Can you work these out from the model? Positions are in its coordinate system, mm. Round coordinates to 2 decimals unless told otherwise and drop trailing zeros. Loops run counter-clockwise (first coordinate to the right, second up) from the corner with the lowest first, then second, coordinate; pieces in that order, holes last. Notation, with made-up numbers: (-37.75, -37.75) -> (-5.75, -37.75) arc R30 ccw to (-5.75, -6.75) -> close; hole circle Ø11 at (47, -12). An arc over 180 degrees is marked (long way). Use a Markdown table: item, result.
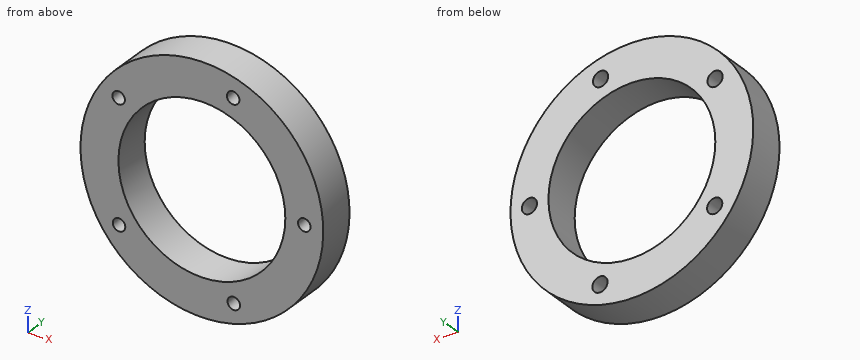
from build123d import *

# Parameters (mm, degrees)
SKETCH1_R                    = 16
SKETCH1_R_2                  = 11
BOSS_EXTRUDE2_DEPTH          = 5
SKETCH2_R                    = 1
CUT_EXTRUDE1_DEPTH           = 5
CUT_EXTRUDE1_DRAFT           = -2
CUT_EXTRUDE1_PROFILE_2_DEPTH = 5
CUT_EXTRUDE1_PROFILE_2_DRAFT = -2
CUT_EXTRUDE1_PROFILE_3_DEPTH = 5
CUT_EXTRUDE1_PROFILE_3_DRAFT = -2
CUT_EXTRUDE1_PROFILE_4_DEPTH = 5
CUT_EXTRUDE1_PROFILE_4_DRAFT = -2
CUT_EXTRUDE1_PROFILE_5_DEPTH = 5
CUT_EXTRUDE1_PROFILE_5_DRAFT = -2


with BuildPart() as part:
    # Sketch1 → Boss-Extrude2 (new body)
    with BuildSketch(Plane(origin=(0, 0, 0), x_dir=(1, 0, 0), z_dir=(0, 1, 0))):
        with Locations(Location((0, 0, 0), (0, 0, 270))):
            Circle(SKETCH1_R)
        with Locations(Location((0, 0, 0), (0, 0, 270))):
            Circle(SKETCH1_R_2, mode=Mode.SUBTRACT)
    extrude(amount=BOSS_EXTRUDE2_DEPTH)


with BuildPart() as cut_extrude1_tool:
    # Sketch2 → Cut-Extrude1 (with draft: the straight prism first)
    with BuildSketch(Plane(origin=(0, 5, 0), x_dir=(1, 0, 0), z_dir=(0, 1, 0))):
        with Locations((-10.918529424, 8.01503688)):
            Circle(SKETCH2_R)
    extrude(amount=-CUT_EXTRUDE1_DEPTH)
    # Cut-Extrude1: the draft: its side faces are tilted about the plane it starts from
    cut_extrude1_sides = [cut_extrude1_tool.faces().sort_by_distance(p)[0] for p in [
        (-11.918529424, 2.5, -8.01503688),
    ]]
    draft(cut_extrude1_sides, Plane(origin=(0, 5, 0), x_dir=(1, 0, 0), z_dir=(0, 1, 0)), CUT_EXTRUDE1_DRAFT)


with BuildPart() as part_1:
    add(part.part)

    # Cut-Extrude1: cut by cut_extrude1_tool
    add(cut_extrude1_tool.part, mode=Mode.SUBTRACT)


with BuildPart() as cut_extrude1_profile_2_tool:
    # Sketch2 → Cut-Extrude1 profile 2 (with draft: the straight prism first)
    with BuildSketch(Plane(origin=(0, 5, 0), x_dir=(1, 0, 0), z_dir=(0, 1, 0))):
        with Locations((-10.966125757, -7.868550431)):
            Circle(SKETCH2_R)
    extrude(amount=-CUT_EXTRUDE1_PROFILE_2_DEPTH)
    # Cut-Extrude1 profile 2: the draft: its side faces are tilted about the plane it starts from
    cut_extrude1_profile_2_sides = [cut_extrude1_profile_2_tool.faces().sort_by_distance(p)[0] for p in [
        (-11.966125757, 2.5, 7.868550431),
    ]]
    draft(cut_extrude1_profile_2_sides, Plane(origin=(0, 5, 0), x_dir=(1, 0, 0), z_dir=(0, 1, 0)), CUT_EXTRUDE1_PROFILE_2_DRAFT)


with BuildPart() as part_2:
    add(part_1.part)

    # Cut-Extrude1 profile 2: cut by cut_extrude1_profile_2_tool
    add(cut_extrude1_profile_2_tool.part, mode=Mode.SUBTRACT)


with BuildPart() as cut_extrude1_profile_3_tool:
    # Sketch2 → Cut-Extrude1 profile 3 (with draft: the straight prism first)
    with BuildSketch(Plane(origin=(0, 5, 0), x_dir=(1, 0, 0), z_dir=(0, 1, 0))):
        with Locations((4.125355383, -12.822115645)):
            Circle(SKETCH2_R)
    extrude(amount=-CUT_EXTRUDE1_PROFILE_3_DEPTH)
    # Cut-Extrude1 profile 3: the draft: its side faces are tilted about the plane it starts from
    cut_extrude1_profile_3_sides = [cut_extrude1_profile_3_tool.faces().sort_by_distance(p)[0] for p in [
        (3.125355383, 2.5, 12.822115645),
    ]]
    draft(cut_extrude1_profile_3_sides, Plane(origin=(0, 5, 0), x_dir=(1, 0, 0), z_dir=(0, 1, 0)), CUT_EXTRUDE1_PROFILE_3_DRAFT)


with BuildPart() as part_3:
    add(part_2.part)

    # Cut-Extrude1 profile 3: cut by cut_extrude1_profile_3_tool
    add(cut_extrude1_profile_3_tool.part, mode=Mode.SUBTRACT)


with BuildPart() as cut_extrude1_profile_4_tool:
    # Sketch2 → Cut-Extrude1 profile 4 (with draft: the straight prism first)
    with BuildSketch(Plane(origin=(0, 5, 0), x_dir=(1, 0, 0), z_dir=(0, 1, 0))):
        with Locations((13.5, 0)):
            Circle(SKETCH2_R)
    extrude(amount=-CUT_EXTRUDE1_PROFILE_4_DEPTH)
    # Cut-Extrude1 profile 4: the draft: its side faces are tilted about the plane it starts from
    cut_extrude1_profile_4_sides = [cut_extrude1_profile_4_tool.faces().sort_by_distance(p)[0] for p in [
        (12.5, 2.5, 0),
    ]]
    draft(cut_extrude1_profile_4_sides, Plane(origin=(0, 5, 0), x_dir=(1, 0, 0), z_dir=(0, 1, 0)), CUT_EXTRUDE1_PROFILE_4_DRAFT)


with BuildPart() as part_4:
    add(part_3.part)

    # Cut-Extrude1 profile 4: cut by cut_extrude1_profile_4_tool
    add(cut_extrude1_profile_4_tool.part, mode=Mode.SUBTRACT)


with BuildPart() as cut_extrude1_profile_5_tool:
    # Sketch2 → Cut-Extrude1 profile 5 (with draft: the straight prism first)
    with BuildSketch(Plane(origin=(0, 5, 0), x_dir=(1, 0, 0), z_dir=(0, 1, 0))):
        with Locations((4.202367867, 12.878068489)):
            Circle(SKETCH2_R)
    extrude(amount=-CUT_EXTRUDE1_PROFILE_5_DEPTH)
    # Cut-Extrude1 profile 5: the draft: its side faces are tilted about the plane it starts from
    cut_extrude1_profile_5_sides = [cut_extrude1_profile_5_tool.faces().sort_by_distance(p)[0] for p in [
        (3.202367867, 2.5, -12.878068489),
    ]]
    draft(cut_extrude1_profile_5_sides, Plane(origin=(0, 5, 0), x_dir=(1, 0, 0), z_dir=(0, 1, 0)), CUT_EXTRUDE1_PROFILE_5_DRAFT)


with BuildPart() as part_5:
    add(part_4.part)

    # Cut-Extrude1 profile 5: cut by cut_extrude1_profile_5_tool
    add(cut_extrude1_profile_5_tool.part, mode=Mode.SUBTRACT)


solid = part_5.part
1. I want a section at B-B (z = 0). Please give me the cut outline in (x, y).
Answer sheet:
| item | result |
|---|---|
| outline | (-16, 0) -> (-11, 0) -> (-11, 5) -> (-16, 5) -> close; (11, 0) -> (12.67, 0) -> (12.5, 5) -> (11, 5) -> close; (14.33, 0) -> (16, 0) -> (16, 5) -> (14.5, 5) -> close |
2. I need wall thicknesses on line 1 (X direction, y = 3, z = 0); line 2 (X direction, y = 1.55, z = -7.5); line 3 (Z direction, x = -11.5, y = 3). Which ranges of each line are inside material? Lowest first, please.
Answer sheet:
| item | result |
|---|---|
| line 1 | x = -16 to -11, 11 to 12.57, 14.43 to 16 |
| line 2 | x = -14.13 to -11.63, -10.21 to -8.05, 8.05 to 14.13 |
| line 3 | z = -11.12 to -8.74, -7.29 to 7.11, 8.63 to 11.12 |
3. Will these pins go through, and if not, where does the flat tip stop? pin 1 Ø3 at (y, z) = (2.5, -9.5) entering from +X; pin 2 Ø2 at (x, y) = (-11, 1.5) entering from +Z; pin 3 Ø1.5 at (x, y) = (-5.5, 4.5) entering from +Z.
Answer sheet:
| item | result |
|---|---|
| pin 1 | stops at x = 13.86 |
| pin 2 | stops at z = 12.49 |
| pin 3 | stops at z = 15.28 |
4. I want a section at C-C (y = 0.95). Please give me the cut outline in (x, z), plus the area to 3 significant figures.
Answer sheet:
| item | result |
|---|---|
| outline | circle Ø32 at (0, 0); hole circle Ø1.72 at (-10.97, 7.87); hole circle Ø1.72 at (-10.92, -8.02); hole circle Ø22 at (0, 0); hole circle Ø1.72 at (4.13, 12.82); hole circle Ø1.72 at (4.2, -12.88); hole circle Ø1.72 at (13.5, 0) |
| area | 413 mm² |
5. I want a section at A-A (x = 0). Please give me the cut outline in (y, z), plus the area to 3 significant figures.
Answer sheet:
| item | result |
|---|---|
| outline | (0, -16) -> (5, -16) -> (5, -11) -> (0, -11) -> close; (0, 11) -> (5, 11) -> (5, 16) -> (0, 16) -> close |
| area | 50.0 mm² |
6. I want a section at D-D (z = 9.5). Please give me the cut outline in (x, y).
Answer sheet:
| item | result |
|---|---|
| outline | (-12.87, 0) -> (-5.55, 0) -> (-5.55, 5) -> (-12.87, 5) -> close; (5.55, 0) -> (12.87, 0) -> (12.87, 5) -> (5.55, 5) -> close |
